from build123d import *

# Parameters (mm, degrees)
EXTRUDE_1_DEPTH     = 100
CUT_EXTRUDE_1_DEPTH = 1027.825534296
CUT_EXTRUDE_2_DEPTH = 100


with BuildPart() as part:
    # 草图1 → 凸台-拉伸1 (new body)
    with BuildSketch(Plane.XY):
        with BuildLine():
            Line((-455.837805225, -595.576943247), (-577.394553286, -754.397461446))
            ThreePointArc((-577.394553286, -754.397461446), (-509.447321611, -801.850002496), (-437.622888206, -843.199980858))
            Line((-437.622888206, -843.199980858), (-345.491753847, -665.684195414))
            ThreePointArc((-345.491753847, -665.684195414), (-402.195253903, -633.039475655), (-455.837805225, -595.576943247))
        make_face()
    extrude(amount=EXTRUDE_1_DEPTH)

    # 草图2 → 切除-拉伸1 (cut, through all)
    with BuildSketch(Plane.XY.offset(100)):
        Polygon((-472.039544491, -766.28120979), (-498.852561418, -808.4838415), (-500.293413788, -812.59937229), (-523.195250823, -798.324469225), (-519.950393134, -795.079611536), (-492.967880598, -752.602438021), align=None)
    extrude(amount=-CUT_EXTRUDE_1_DEPTH, mode=Mode.SUBTRACT)

    # 草图4 → 切除-旋转1 (revolve, cut)
    with BuildSketch(Plane(origin=(-29.5994078, 18.802248971, 0), x_dir=(0, 0, -1), z_dir=(0.8440969905384018, -0.5361905170403645, 0)), mode=Mode.PRIVATE) as cut_revolve_1_sk:
        Polygon((-100, -802.210780827), (-100, -797.210780827), (-50.759612349, -788.528371944), (0, -788.528371944), (0, -802.210780827), align=None)
    cut_revolve_1 = revolve(cut_revolve_1_sk.sketch.rotate(Axis((-459.737221147, -658.341456902, 100), (0, 0, -1)), 57.57531458), axis=Axis((-459.737221147, -658.341456902, 100), (0, 0, -1)), mode=Mode.SUBTRACT)

    # 镜向1: 切除-旋转1 across plane
    add(cut_revolve_1.mirror(Plane(origin=(0, 0, 0), x_dir=(0, 0, 1), z_dir=(-0.8440526342067589, 0.5362603385377582, 0))), mode=Mode.SUBTRACT)

    # 草图6 → 切除-拉伸2 (cut)
    with BuildSketch(Plane.XY.offset(100)):
        with BuildLine():
            Line((-501.421585748, -655.134637572), (-516.607469043, -674.975821978))
            ThreePointArc((-516.607469043, -674.975821978), (-496.522608458, -689.884727049), (-476.007750242, -704.196179367))
            Line((-476.007750242, -704.196179367), (-462.015311929, -683.496050861))
            ThreePointArc((-462.015311929, -683.496050861), (-481.927127678, -669.605289411), (-501.421585748, -655.134637572))
        make_face()
        with BuildLine():
            Line((-380.040929232, -732.252614955), (-391.550719321, -754.429368148))
            ThreePointArc((-391.550719321, -754.429368148), (-413.579890996, -742.581518144), (-435.250907035, -730.090600714))
            Line((-435.250907035, -730.090600714), (-422.456532439, -708.62929533))
            ThreePointArc((-422.456532439, -708.62929533), (-401.422544589, -720.753037243), (-380.040929232, -732.252614955))
        make_face()
    extrude(amount=-CUT_EXTRUDE_2_DEPTH, mode=Mode.SUBTRACT)


solid = part.part
Model file for the job. Use its own axes, mm. A direction names the side the tool comes from. Give positions to 0.01 mm unless a question says otherwise; leave off trailing zeros. Loops run counter-clockwise (first coordinate to the right, second up) from the corner with the lowest first, then second, coordinate; pieces in that order, holes last. Notation, with made-up numbers: (-3, 50) - (51, 50) arc R4 ccw to (51, 56) - close; hole circle Ø9 at (83, -38). An arc over 180 degrees is marked (long way). Use one line per item in the form item = value.
(1) Drill centre lines: L1, parallel to Y at x = -481, z = 59.5; L2, parallel to Y at x = -413, z = 16.5; L3, parallel to X at y = -700, z = 19. Where is each one in solid material? Low to high.
Determined:
L1 = -819.23 to -780.38, -760.42 to -700.8, -670.27 to -628.45
L2 = -795.76 to -742.9, -714.18 to -701.78, -689.98 to -626.04
L3 = -535.76 to -482.16, -473.17 to -413.7, -387.61 to -363.3
(2) Cut at D-D (z = 20). Give the cut face in (x, y).
Determined:
outline = (-577.39, -754.4) arc R950 ccw to (-519.95, -795.08) - (-492.97, -752.6) - (-472.04, -766.28) - (-498.85, -808.48) arc R950 ccw to (-437.62, -843.2) - (-391.55, -754.43) arc R849.99 cw to (-435.25, -730.09) - (-422.46, -708.63) arc R825 ccw to (-380.04, -732.25) - (-345.49, -665.68) arc R750 cw to (-455.84, -595.58) - (-501.42, -655.13) arc R825 ccw to (-462.02, -683.5) - (-476.01, -704.2) arc R849.99 cw to (-516.61, -674.98) - close; hole circle Ø27.36 at (-459.74, -658.34); hole circle Ø27.36 at (-400.65, -695.88)
(3) Cut at A-A (x = -489). Give the cut face in (y, z), then the cut area to 3 significant figures.
Determined:
outline = (-814.48, 0) - (-792.98, 0) - (-792.98, 100) - (-814.48, 100) - close; (-755.2, 0) - (-695.24, 0) - (-695.24, 100) - (-755.2, 100) - close; (-664.46, 0) - (-638.91, 0) - (-638.91, 100) - (-664.46, 100) - close
area = 10,700 mm^2
(4) Cut at C-C (y = -758). Give the cut face in (x, z), then the cut area to 3 significant figures.
Determined:
outline = (-572.66, 0) - (-496.4, 0) - (-496.4, 100) - (-572.66, 100) - close; (-484.71, 0) - (-393.4, 0) - (-393.4, 100) - (-484.71, 100) - close
area = 16,800 mm^2
(5) 3-axis set-ups, long thin cutter, end or side, ignore diameter. For faces 1 (the face through (-496.81, -689.68, 50.7)), 2 (the face through (-412.178, -703.256, 25.024)), 3 (the face through (-463, -718, 100)): which of +Z, -Z, +X, -X, +Y, -Y reach the whole face in a straight line?
Determined:
face_1 = +Z, -Z
face_2 = -Z
face_3 = +Z, +X, -X, +Y, -Y
(6) Drop flat-ended pins along their axis: P1, Ø6, axis at y = -771, z = 46, coming from the +X side; P2, Ø10, axis at x = -374, z = 79.5, coming from the +Y side; P3, Ø10, axis at y = -628, z = 26.5, coming from the +X side; P4, Ø12, axis at x = -438.5, y = -693.5, coming from the -Z side. Give the stop position or say it passes through.
Determined:
P1 = -398.59
P2 = -647.19
P3 = -402.26
P4 = 0
(7) Cut at B-B (z = 87.5). Give the cut face in (x, y), then the cut area to 3 significant figures.
Determined:
outline = (-577.39, -754.4) arc R950 ccw to (-519.95, -795.08) - (-492.97, -752.6) - (-472.04, -766.28) - (-498.85, -808.48) arc R950 ccw to (-437.62, -843.2) - (-391.55, -754.43) arc R849.99 cw to (-435.25, -730.09) - (-422.46, -708.63) arc R825 ccw to (-380.04, -732.25) - (-345.49, -665.68) arc R750 cw to (-455.84, -595.58) - (-501.42, -655.13) arc R825 ccw to (-462.02, -683.5) - (-476.01, -704.2) arc R849.99 cw to (-516.61, -674.98) - close; hole circle Ø14.41 at (-459.74, -658.34); hole circle Ø14.41 at (-400.65, -695.88)
area = 25,600 mm^2
(8) Pull direction X, two halves, no side cores. Call faces 4 (the face through (-463, -718, 0)), 5 (the face through (-549.452, -774.986, 49.3)), 6 (the face through (-394.946, -688.409, 75.035)), 7 (the face through (-451.052, -654.74, 75.035)): pulls with the +X half, pulls with the -X half, needs draft (parallel to the pull), parting line crosses it, or undercut.
Determined:
face_4 = needs draft
face_5 = pulls with the -X half
face_6 = undercut
face_7 = undercut
